Verification items for the finished model (mm, model axes). A direction names the side the tool comes from. Coordinates: 2 decimals unless noted, no trailing zeros. Order: outer loops, then holes, each group sorted by start corner. A loop starts at its lowest first (then second) coordinate and runs counter-clockwise, first axis right, second up. Notation, with made-up numbers: M -19.5,-5.5 L 19.5,-5.5 A19 ccw 19.5,-0.5 Z; hole C -14.75,79 d7. An arc over 180 degrees is marked long. Return JSON: item names as keys, results as strings.
```python
from build123d import *

# Parameters (mm, degrees)
SKETCH1_R               = 20
BOSS_EXTRUDE1_DEPTH     = 40
SKETCH2_W               = 30
SKETCH2_H               = 2
CUT_EXTRUDE1_DEPTH      = 40
CUT_EXTRUDE1_DEPTH_BACK = 40
SKETCH3_W               = 10
SKETCH3_H               = 20
CUT_EXTRUDE2_DEPTH      = 40
CUT_EXTRUDE2_DEPTH_BACK = 40
SKETCH4_W               = 30
SKETCH4_H               = 20
CUT_EXTRUDE4_DEPTH      = 40


with BuildPart() as part:
    # Sketch1 → Boss-Extrude1 (new body)
    with BuildSketch(Plane.XY):
        Circle(SKETCH1_R)
    extrude(amount=BOSS_EXTRUDE1_DEPTH)

    # Sketch2 → Cut-Extrude1 (cut, two sides)
    with BuildSketch(Plane(origin=(0, 0, 0), x_dir=(0, 0, -1), z_dir=(1, 0, 0))) as cut_extrude1_sk:
        with Locations((-25, 19)):
            Rectangle(SKETCH2_W, SKETCH2_H)
    extrude(amount=CUT_EXTRUDE1_DEPTH, mode=Mode.SUBTRACT)
    extrude(cut_extrude1_sk.sketch, amount=-CUT_EXTRUDE1_DEPTH_BACK, mode=Mode.SUBTRACT)

    # Sketch3 → Cut-Extrude2 (cut, two sides)
    with BuildSketch(Plane(origin=(0, 0, 0), x_dir=(0, 0, -1), z_dir=(1, 0, 0))) as cut_extrude2_sk:
        with Locations((-35, 10)):
            Rectangle(SKETCH3_W, SKETCH3_H)
    extrude(amount=CUT_EXTRUDE2_DEPTH, mode=Mode.SUBTRACT)
    extrude(cut_extrude2_sk.sketch, amount=-CUT_EXTRUDE2_DEPTH_BACK, mode=Mode.SUBTRACT)

    # Sketch4 → Cut-Extrude4 (cut)
    with BuildSketch(Plane(origin=(0, 0, 0), x_dir=(1, 0, 0), z_dir=(0, 1, 0))):
        with Locations((-5, -20)):
            Rectangle(SKETCH4_W, SKETCH4_H)
    extrude(amount=CUT_EXTRUDE4_DEPTH, mode=Mode.SUBTRACT)


solid = part.part
```
Q1. Cross-section at A-A, the plane x = 0. Record the boundary of the cut face in (y, z).
Values:
{"outline": "M -20,0 L 20,0 L 20,10 L 0,10 L 0,40 L -20,40 Z"}
Q2. Go/stop test with flat-tipped pins: pin 1 (1 mm diameter, centred on x = -4, y = 12, fed in from +Z); pin 2 (10 mm diameter, centred on x = -2.5, z = 27, fed in from -Y); pin 3 (5 mm diameter, centred on y = 8, z = 15.5, fed in from -X). Record where each tip stops, or that it passes through.
Values:
{"pin 1": "z = 10", "pin 2": "y = -20", "pin 3": "x = 10"}
Q3. Material ranges on line 1 along Y through (x, z) = (0, 6.5); line 2 along Z through (x, y) = (2.5, 10); line 3 along Z through (x, y) = (11.5, 7.5), recorded low to high.
Values:
{"line 1": "-20 to 20", "line 2": "0 to 10", "line 3": "0 to 30"}
Q4. Cross-section at D-D, the plane y = -9. Record the boundary of the cut face in (x, z).
Values:
{"outline": "M -17.86,0 L 17.86,0 L 17.86,40 L -17.86,40 Z"}
Q5. Cross-section at C-C, the plane y = 3.5. Record the boundary of the cut face in (x, z).
Values:
{"outline": "M -19.69,0 L 19.69,0 L 19.69,30 L 10,30 L 10,10 L -19.69,10 Z"}
Q6. Tool access check on faces 1 (the face through (0, -8, 40)), 2 (the face through (-5, 10, 10)), 3 (the face through (14, 7, 30)). Record the directions out of +Z, -Z, +X, -X, +Y, -Y that give a thin tool (end or side, any length) a straight path to the whole face; none if there is none.
Values:
{"face 1": "+Z, +X, -X, +Y, -Y", "face 2": "+Z, -X, +Y", "face 3": "+Z, +X, -X, +Y"}
Q7. Cross-section at B-B, the plane z = 11. Record the boundary of the cut face in (x, y).
Values:
{"outline": "M -20,0 A20 ccw long 10,17.32 L 10,0 Z"}
